Check sheet for the modelled part. Datum: model origin and axes. Units: mm. Round coordinates to 2 decimals unless told otherwise and drop trailing zeros. Order: outer loops, then holes, each group sorted by start corner. A loop starts at its lowest first (then second) coordinate and runs counter-clockwise, first axis right, second up. Notation, with made-up numbers: (-2, 47) -> (42, 47) arc R33 ccw to (42, 76) -> close; hole circle Ø10 at (-23, -40). An arc over 180 degrees is marked (long way). Use CSV: the item, a comma, the result in double quotes.
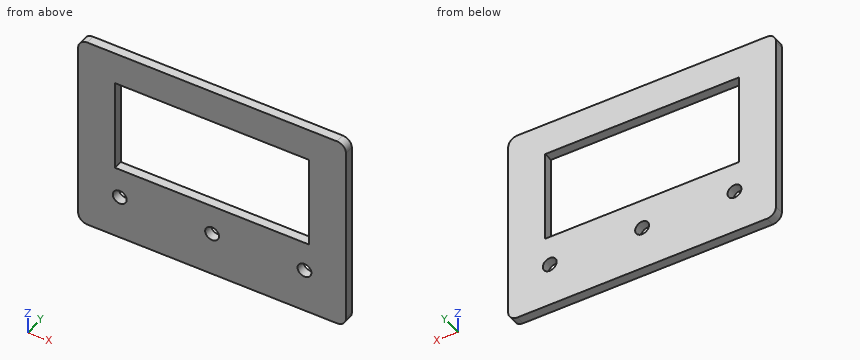
```python
from build123d import *

# Parameters (mm, degrees)
SKETCH1_W           = 58
SKETCH1_H           = 43
SKETCH1_R           = 1.5
SKETCH1_W_2         = 42
SKETCH1_H_2         = 20
BOSS_EXTRUDE1_DEPTH = 2
FILLET1_R           = 2


with BuildPart() as part:
    # Sketch1 → Boss-Extrude1 (new body)
    with BuildSketch(Plane(origin=(0, 0, 0), x_dir=(1, 0, 0), z_dir=(0, 1, 0))):
        Rectangle(SKETCH1_W, SKETCH1_H)
        with Locations(Location((0, 12, 0), (0, 0, 270))):
            Circle(SKETCH1_R, mode=Mode.SUBTRACT)
        with Locations(Location((20, 12, 0), (0, 0, 270))):
            Circle(SKETCH1_R, mode=Mode.SUBTRACT)
        with Locations(Location((-20, 12, 0), (0, 0, 270))):
            Circle(SKETCH1_R, mode=Mode.SUBTRACT)
        with Locations((0, -4.5)):
            Rectangle(SKETCH1_W_2, SKETCH1_H_2, mode=Mode.SUBTRACT)
    extrude(amount=BOSS_EXTRUDE1_DEPTH)

    # Fillet1
    fillet1_edges = [part.edges().sort_by_distance(p)[0] for p in [
        (29, 1, 21.5),
        (-29, 1, 21.5),
        (-29, 1, -21.5),
        (29, 1, -21.5),
    ]]
    fillet(fillet1_edges, radius=FILLET1_R)


solid = part.part
```
Q1. Sectioned sample at B-B, the plane x = 5. Enter the section's corners in (y, z).
Result sheet:
outline,"(0, -21.5) -> (2, -21.5) -> (2, -5.5) -> (0, -5.5) -> close; (0, 14.5) -> (2, 14.5) -> (2, 21.5) -> (0, 21.5) -> close"
Q2. Sectioned sample at C-C, the plane y = 1.65. Enter the section's corners in (x, z), then the cut area to 3 significant figures.
Result sheet:
outline,"(-29, -19.5) arc R2 ccw to (-27, -21.5) -> (27, -21.5) arc R2 ccw to (29, -19.5) -> (29, 19.5) arc R2 ccw to (27, 21.5) -> (-27, 21.5) arc R2 ccw to (-29, 19.5) -> close; hole circle Ø3 at (-20, -12); hole (-21, -5.5) -> (21, -5.5) -> (21, 14.5) -> (-21, 14.5) -> close; hole circle Ø3 at (0, -12); hole circle Ø3 at (20, -12)"
area,"1,630 mm^2"
Q3. Go/stop test with a flat-tipped pin: pin 1 (8 mm diameter, centred on x = -4, z = 0.5, fed in from -Y). Record where the tip stops, or that it passes through.
Result sheet:
pin 1,"passes through"
Q4. Scan lines: L1, parallel to X at y = 1.25, z = -12; L2, parallel to Z at x = -7.5, y = 0.2; L3, parallel to X at y = 1.3, z = 8. Record each from-to range of solid material in increasing order.
Result sheet:
L1,"x = -29 to -21.5, -18.5 to -1.5, 1.5 to 18.5, 21.5 to 29"
L2,"z = -21.5 to -5.5, 14.5 to 21.5"
L3,"x = -29 to -21, 21 to 29"
Q5. Sectioned sample at A-A, the plane z = -12. Enter the section's corners in (x, y).
Result sheet:
outline,"(-29, 0) -> (-21.5, 0) -> (-21.5, 2) -> (-29, 2) -> close; (-18.5, 0) -> (-1.5, 0) -> (-1.5, 2) -> (-18.5, 2) -> close; (1.5, 0) -> (18.5, 0) -> (18.5, 2) -> (1.5, 2) -> close; (21.5, 0) -> (29, 0) -> (29, 2) -> (21.5, 2) -> close"
Q6. Sectioned sample at D-D, the plane z = 7. Enter the section's corners in (x, y).
Result sheet:
outline,"(-29, 0) -> (-21, 0) -> (-21, 2) -> (-29, 2) -> close; (21, 0) -> (29, 0) -> (29, 2) -> (21, 2) -> close"
